Could you check a few things on this model? Use its own coordinates, in mm. A direction names the side the tool comes from. Give positions to 0.01 mm unless a question says otherwise; leave off trailing zeros. Order: outer loops, then holes, each group sorted by start corner. A loop starts at its lowest first (then second) coordinate and runs counter-clockwise, first axis right, second up. Notation, with made-up numbers: (-6, -12) -> (14, -12) arc R28 cw to (14, 11) -> close; hole circle Ø4 at (-20.75, -21.5). An arc over 180 degrees is marked (long way). Write each question's results on one line, items separated by ' | '.
Autodesk Inventor part; units mm, degrees
ref_plane "YZ Plane" through (0, 0, 0) normal (1, 0, 0) x (0, 1, 0)
ref_plane "XZ Plane" through (0, 0, 0) normal (0, 1, 0) x (-1, 0, 0)
ref_plane "XY Plane" through (0, 0, 0) normal (0, 0, 1) x (1, 0, 0)
sketch "Sketch1" plane through (0, 0, 0) normal (0, 1, 0) x (-1, 0, 0)
  line L0 (15.75, 0) -> (-15.75, 0) construction
  line L1 (15.75, 40) -> (-15.75, 40)
  line L2 (-15.75, 40) -> (-15.75, 24)
  line L3 (15.75, 24) -> (-15.75, 24)
  line L4 (15.75, 24) -> (15.75, 40)
  line L5 (3.9375, 0) -> (-3.9375, 0)
  line L6 (-3.9375, 0) -> (-3.9375, 24)
  line L7 (-3.9375, 24) -> (3.9375, 24)
  line L8 (3.9375, 24) -> (3.9375, 0)
  line L9 (3.9375, 0) -> (-3.9375, 24) construction
  line L10 (-3.9375, 0) -> (3.9375, 24) construction
  point P0 (0, 12)
  point P1 (0, 24)
  point P2 (0, 0)
  point P3 (0, 0)
  dimension "Thickness" = 31.5
  dimension "DiamExt" = 80
  dimension "PipeDiameter" = 48
  dimension "d8" = 7.875
revolve "Revolution1" add sketch "Sketch1" angle 360 about axis through (-15.75, 0, 0) along (1, 0, 0)
sketch "Sketch5" plane through (-3.9375, 0, 0) normal (-1, 0, 0) x (0, 0, 1)
  circle A0 centre (0, 0) radius 40
  line L0 (0, 0) -> (33.9411, 33.9411) construction
  line L1 (0, 0) -> (48, 0) construction
  circle A1 centre (33.9411, 33.9411) radius 8 construction
  circle A2 centre (0, 0) radius 40
  line L2 (40, 0) -> (40, 25.9411)
  line L3 (40, 25.9411) -> (30.4476, 25.9411)
  point P0 (0, 0)
  dimension "d18" = 45
  dimension "d19" = 16
extrude "Extrusion1" add sketch "Sketch5" against normal up to surface (7.875 mm away) from surface at 0 contours A0 L3 L2
pattern_circular "Circular Pattern1" count 4 over 360 about axis through (0, 0, 0) along (-1, 0, 0) of "Extrusion1"
equation "\"d8\" = 0.25 * Thickness"
properties part number "CHECK VALVE DISK WAFER 316L DN40" material "304L"
Q1. I need wall thicknesses on line 1 along Z through (x, y) = (10, 0); line 2 along X through (y, z) = (-15.5, -9). Which ranges of each line are inside material? Lowest first, please.
Here are the results:
line 1: z = -40 to -24, 24 to 40 | line 2: x = -3.94 to 3.94
Q2. For faces 4 (the flat face through (3.938, 0, 0)), 5 (the flat face through (-3.938, -37, 20)), 6 (the flat face through (3.938, -37, 20)), which set-ups out of +Z, -Z, +X, -X, +Y, -Y let a thin tool reach every point of the face, with its end or its side?
Here are the results:
face 4: +X | face 5: +Z, -X, -Y | face 6: +Z, +X, -Y
Q3. Suppose I cut it at B-B on y = 6.5. Please give me the cut outline in (x, z).
Here are the results:
outline: (-15.75, -39.47) -> (15.75, -39.47) -> (15.75, -23.1) -> (3.94, -23.1) -> (3.94, 23.1) -> (15.75, 23.1) -> (15.75, 39.47) -> (3.94, 39.47) -> (3.94, 40) -> (-3.94, 40) -> (-3.94, 39.47) -> (-15.75, 39.47) -> (-15.75, 23.1) -> (-3.94, 23.1) -> (-3.94, -23.1) -> (-15.75, -23.1) -> close
Q4. I'm going to push flat-ended pins straight in: pin 1 Ø1.5 at (x, z) = (3.5, -19) entering from -Y; pin 2 Ø4 at (x, z) = (0, 37) entering from +Y; pin 3 Ø4 at (y, z) = (-3, -13) entering from +X. Where does each tip first touch, or does it pass through?
Here are the results:
pin 1: stops at y = -35.59 | pin 2: stops at y = 25.94 | pin 3: stops at x = 3.94
Q5. Thinking about a two-plate mould opening in Z: for faces 1 (the flat face through (3.938, -20, -37)), 2 (the cylindrical face through (-9.761, -1.055, -23.977)), 3 (the flat face through (0, -13, -40)), which applies, +Z half, -Z half, draft (parallel to the pull), parting line (faces both ways), or undercut?
Here are the results:
face 1: draft | face 2: undercut | face 3: -Z half
Q6. Suppose I cut it at D-D on y = -32. Please give me the cut outline in (x, z).
Here are the results:
outline: (-15.75, -24) -> (15.75, -24) -> (15.75, 24) -> (3.94, 24) -> (3.94, 25.94) -> (-3.94, 25.94) -> (-3.94, 24) -> (-15.75, 24) -> close
Q7. Suppose I cut it at A-A on x = -10. Please give me the cut outline in (y, z), and give its area (3 significant figures).
Here are the results:
outline: circle Ø80 at (0, 0); hole circle Ø48 at (0, 0) | area: 3,220 mm²
Q8. Suppose I cut it at C-C on z = 22. Please give me the cut outline in (x, y), and give its area (3 significant figures).
Here are the results:
outline: (-15.75, -33.41) -> (-3.94, -33.41) -> (-3.94, -40) -> (3.94, -40) -> (3.94, -33.41) -> (15.75, -33.41) -> (15.75, -9.59) -> (3.94, -9.59) -> (3.94, 9.59) -> (15.75, 9.59) -> (15.75, 33.41) -> (-15.75, 33.41) -> (-15.75, 9.59) -> (-3.94, 9.59) -> (-3.94, -9.59) -> (-15.75, -9.59) -> close | area: 1,700 mm²
